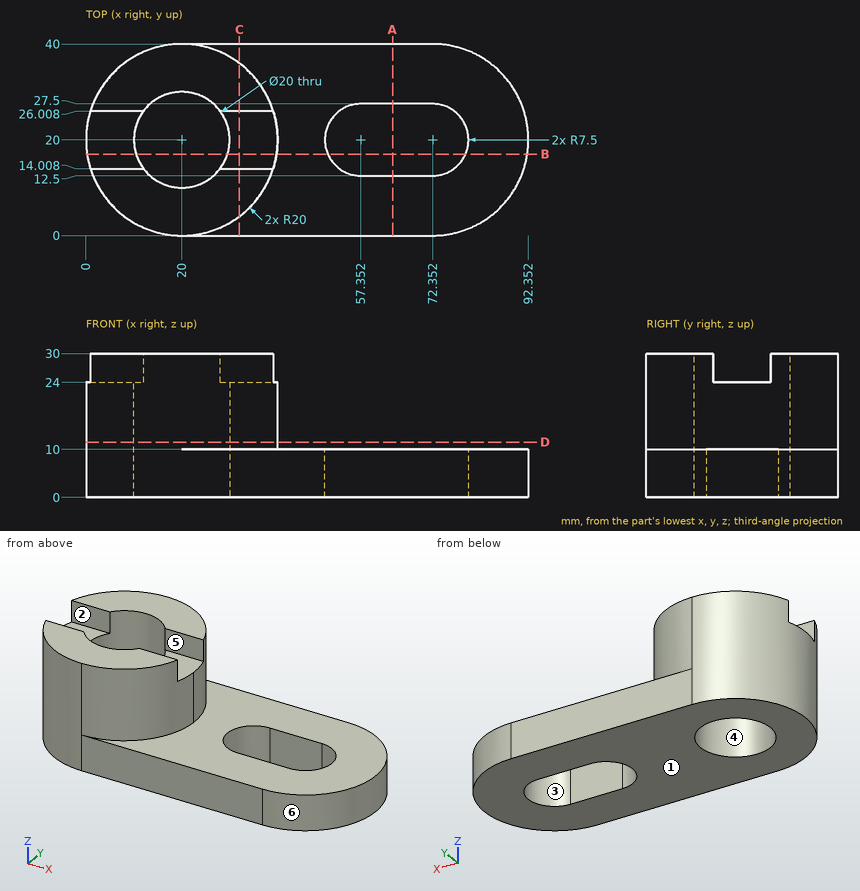
Here's the drawing with two shaded views (mm, measured from the low corner). I have some questions. A direction names the side the tool comes from. Coordinates: 2 decimals unless noted, no trailing zeros. Write each loop counter-clockwise with the first axis right and the second up, starting at its lowest first coordinate (ties: lowest second). Pieces come first, ordered by that corner, then holes. Notation, with made-up numbers: (62.25, -9) - (71.25, -9) arc R32 ccw to (71.25, 23) - close; hole circle Ø10 at (39.25, 36). An arc over 180 degrees is marked (long way). Return JSON: item names as keys, results as strings.
Q1. If we section it at A-A (x = 64): Please give me the cut outline in (y, z).
Computed values:
{"outline": "(0, 0) - (12.5, 0) - (12.5, 10) - (0, 10) - close; (27.5, 0) - (40, 0) - (40, 10) - (27.5, 10) - close"}
Q2. If we section it at C-C (x = 32): Please give me the cut outline in (y, z), then the cut area to 3 significant figures.
Computed values:
{"outline": "(0, 0) - (40, 0) - (40, 10) - (36, 10) - (36, 30) - (26.01, 30) - (26.01, 24) - (14.01, 24) - (14.01, 30) - (4, 30) - (4, 10) - (0, 10) - close", "area": "968 mm2"}
Q3. On a 3-axis mill with a long thin cutter (end or side, diameter ignored), from which of +Z, -Z, +X, -X, +Y, -Y can I reach the whole of each face in a straight line? I mean the marked faces 1, 2 and 3. Say none if no direction works.
Computed values:
{"face 1": "-Z, +X, -X, +Y, -Y", "face 2": "+Z, +X, -X", "face 3": "+Z, -Z"}
Q4. If we section it at D-D (z = 11.5): Please give me the cut outline in (x, y).
Computed values:
{"outline": "circle Ø40 at (20, 20); hole circle Ø20 at (20, 20)"}
Q5. I'm going to push flat-ended pins straight in: pin 1 Ø6 at (y, z) = (12, 22.5) entering from +X (1 decimal); pin 2 Ø6 at (y, z) = (26.5, 10) entering from -X; pin 3 Ø3 at (x, z) = (4.5, 26.5) entering from +Y. Where does each tip first touch, or does it pass through?
Computed values:
{"pin 1": "stops at x = 39.4", "pin 2": "stops at x = 0.31", "pin 3": "stops at y = 34.28"}
Q6. Please list where these lines run through material, in increasing order: L1, parallel to X at y = 20, z = 19.75; L2, parallel to Y at x = 63, z = 2.75; L3, parallel to X at y = 16, z = 8.75 (1 decimal). Write a range as from..to.
Computed values:
{"L1": "x = 0..10, 30..40", "L2": "y = 0..12.5, 27.5..40", "L3": "x = 0.4..10.8, 29.2..51, 78.7..91.9"}
Q7. Thinking about a two-plate mould opening in X: for the marked faces 4, 5 and 6, which applies, +X half, -X half, draft (parallel to the pull), parting line (faces both ways), or undercut?
Computed values:
{"face 4": "undercut", "face 5": "draft", "face 6": "+X half"}
Q8. If we section it at B-B (y = 17): Please give me the cut outline in (x, z).
Computed values:
{"outline": "(0.23, 0) - (10.46, 0) - (10.46, 24) - (0.23, 24) - close; (29.54, 0) - (50.48, 0) - (50.48, 10) - (39.77, 10) - (39.77, 24) - (29.54, 24) - close; (79.23, 0) - (92.13, 0) - (92.13, 10) - (79.23, 10) - close"}
